from build123d import *

# Parameters (mm, degrees)
SWEEP1_PROFILE_R        = 5
CUT_EXTRUDE1_DEPTH      = 61.415230017
CUT_EXTRUDE1_DEPTH_BACK = 61.415230017
CUT_EXTRUDE3_DEPTH      = 61.415230017
CUT_EXTRUDE3_DEPTH_BACK = 61.415230017


with BuildPart() as part:
    # Sweep1: sweep along a path in Sketch2
    with BuildLine(Plane.XY) as sweep1_path:
        Line((40, -30), (40, 0))
        Line((40, 0), (40, 15))
        ThreePointArc((40, 15), (20, 35), (0, 15))
        Line((0, 15), (0, 0))
        Line((0, 0), (0, -30))
    # Sweep1 profile (on start of the path) → Sweep1 (sweep)
    with BuildSketch(Plane(origin=(40, -30, 0), x_dir=(1, 0, 0), z_dir=(0, 1, 0))):
        Circle(SWEEP1_PROFILE_R)
    sweep(path=sweep1_path.line)

    # Sketch14 → Cut-Extrude1 (cut, two sides: drawn at the far end of the back side and taken through both)
    with BuildSketch(Plane.XY.offset(-CUT_EXTRUDE1_DEPTH_BACK)):
        with BuildLine():
            Line((6, -5), (34, -5))
            ThreePointArc((34, -5), (40, -11), (34, -17))
            Line((34, -17), (6, -17))
            ThreePointArc((6, -17), (0, -11), (6, -5))
        make_face()
    extrude(amount=CUT_EXTRUDE1_DEPTH + CUT_EXTRUDE1_DEPTH_BACK, mode=Mode.SUBTRACT)

    # Sketch22 → Cut-Extrude3 (cut, two sides: drawn at the far end of the back side and taken through both)
    with BuildSketch(Plane.XY.offset(-CUT_EXTRUDE3_DEPTH_BACK)):
        Polygon((-5, -30), (5, -21.916079783), (5, -30), align=None)
        Polygon((35, -30), (45, -30), (35, -21.916079783), align=None)
    extrude(amount=CUT_EXTRUDE3_DEPTH + CUT_EXTRUDE3_DEPTH_BACK, mode=Mode.SUBTRACT)


solid = part.part
Read the model definition and answer for the solid it produces. Units are mm, in the model's axes. A direction names the side the tool comes from. Round coordinates to 2 decimals unless told otherwise and drop trailing zeros. Write each loop counter-clockwise with the first axis right and the second up, starting at its lowest first coordinate (ties: lowest second). Pieces come first, ordered by that corner, then holes.
Q1. Flat-ended cylindrical pins translate along their axes: P1, Ø3, axis at x = 3.5, y = -9, coming from the +Z side; P2, Ø1.5, axis at x = 29, z = -2, coming from the -Y side; P3, Ø1, axis at y = 17, z = 0.5, coming from the +X side; P4, Ø3, axis at x = 30, z = 2.5, coming from the +Y side. Find the tip coordinate at first contact, or state that the pin passes through.
Values:
P1: passes through
P2: stops at y = 26.84
P3: stops at x = 44.94
P4: stops at y = 38.12
Q2. Find section C-C on z = 3.25. Determine the outline of the cut face in (x, y), and give its area (3 significant figures).
Values:
outline: (-3.8, -29.03) - (3.8, -22.89) - (3.8, -16.58) arc R6 cw to (3.8, -5.42) - (3.8, 15) arc R16.2 cw to (36.2, 15) - (36.2, -5.42) arc R6 cw to (36.2, -16.58) - (36.2, -22.89) - (43.8, -29.03) - (43.8, 15) arc R23.8 ccw to (-3.8, 15) - close
area: 1,040 mm2
Q3. The mould has two halves that part along Y. Classify faces 1 (the face through (0, -11, 0)), 2 (the face through (44.619, -7.185, 1.915)), 3 (the face through (40.07, -26.015, -0.07)), 4 (the face through (40, -11, 0)): released by +Y, released by -Y, zero draft, split by the parting line, or undercut.
Values:
face 1: undercut
face 2: zero draft
face 3: released by -Y
face 4: undercut
Q4. A tool of negligible diameter and unlimited length cuts with its end or side. For faces 5 (the face through (-0.07, -26.015, -0.07)), 6 (the face through (-4.77, -7.82, -1.5)), from which of +Z, -Z, +X, -X, +Y, -Y can it reach the whole face along a straight path? Write none if from no direction.
Values:
face 5: +Z, -Z, -Y
face 6: -Y
Q5. Find section D-D on y = -24. Determine the outline of the cut face in (x, z), and give its area (3 significant figures).
Values:
outline: (2.42, -4.37) - (2.42, 4.37) arc R5 ccw (long way) to start; (37.58, -4.37) arc R5 ccw (long way) to (37.58, 4.37) - close
area: 125 mm2
Q6. Straight lines are drawn through the part: line 1 (X direction, y = -17, z = -0.25); line 2 (X direction, y = 28, z = -3.5); line 3 (Y direction, x = 15, z = -1.75). For each, find the intervals that lie inside material, in ascending order.
Values:
line 1: x = -4.99 to 4.99, 35.01 to 44.99
line 2: x = 0.34 to 9.95, 30.05 to 39.66
line 3: y = 29.48 to 39.17
Q7. Find section B-B on y = -1. Determine the outline of the cut face in (x, z).
Values:
outline: circle Ø10 at (0, 0); circle Ø10 at (40, 0)
Q8. Find section A-A on z = 0. Determine the outline of the cut face in (x, y), and give its area (3 significant figures).
Values:
outline: (-5, -30) - (5, -21.92) - (5, -16.92) arc R6 cw to (5, -5.08) - (5, 15) arc R15 cw to (35, 15) - (35, -5.08) arc R6 cw to (35, -16.92) - (35, -21.92) - (45, -30) - (45, 15) arc R25 ccw to (-5, 15) - close
area: 1,360 mm2
